Part print with two shaded views. Sizes in mm from the minimum x, y, z corner. Give positions to 0.01 mm unless a question says otherwise; leave off trailing zeros. Order: outer loops, then holes, each group sorted by start corner. A loop starts at its lowest first (then second) coordinate and runs counter-clockwise, first axis right, second up. Notation, with made-up numbers: M 25,-3 L 48,-3 A25 ccw 48,29 Z; hole C 78,78 d5. An arc over 180 degrees is marked long. Return JSON: item names as keys, results as strings.
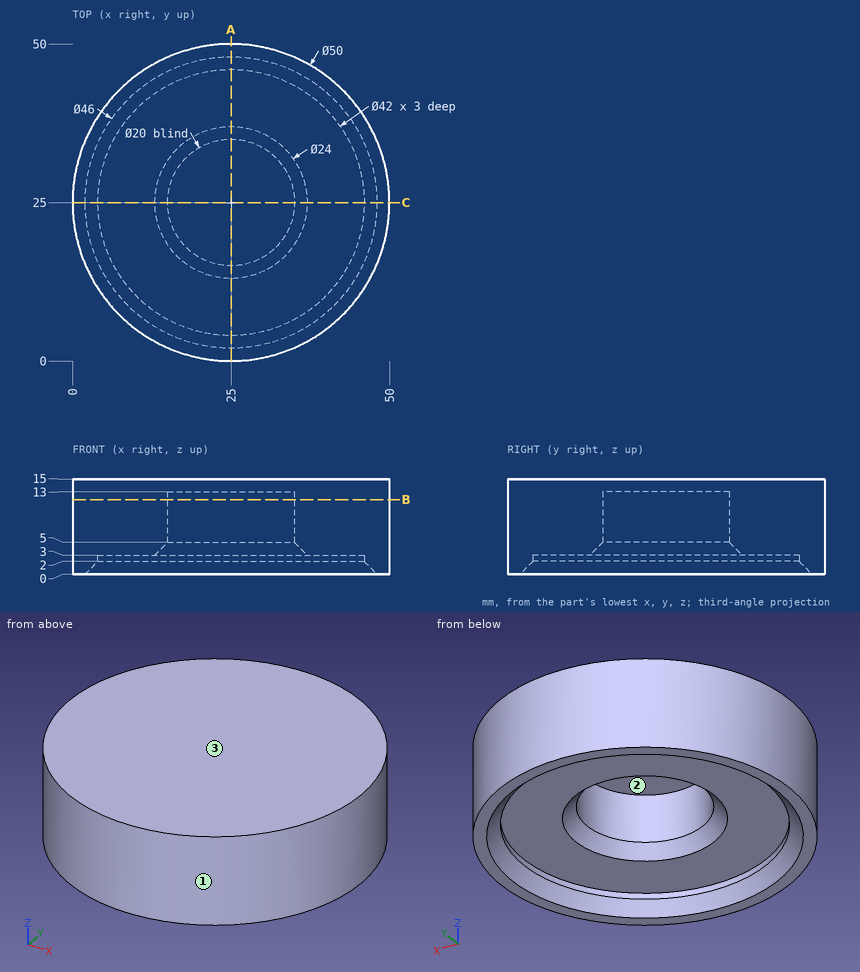
Q1. Probe line 1 along Y through (x, z) = (25, 9.25); line 2 along Z through (x, y) = (12.5, 35); line 3 along Y through (x, z) = (25, 2.7). List the from-to ranges inside material, lowest first.
Established:
{"line 1": "y = 0 to 15, 35 to 50", "line 2": "z = 3 to 15", "line 3": "y = 0 to 4, 46 to 50"}
Q2. Pin check, flat tips, straight feed: pin 1 (6 mm diameter, centred on y = 45, z = 6, fed in from -X); pin 2 (1.5 mm diameter, centred on x = 40, z = 10, fed in from +Y); pin 3 (6 mm diameter, centred on y = 30.5, z = 1.5, fed in from -X). Stop position of each tip, or through.
Established:
{"pin 1": "stops at x = 6.67", "pin 2": "stops at y = 45.54", "pin 3": "stops at x = 0.13"}
Q3. Band-saw the part on A-A (x = 25). Give the cut face in (y, z).
Established:
{"outline": "M 0,0 L 2,0 L 4,2 L 4,3 L 13,3 L 15,5 L 15,13 L 35,13 L 35,5 L 37,3 L 46,3 L 46,2 L 48,0 L 50,0 L 50,15 L 0,15 Z"}
Q4. Two-plate mould, pull along X, no slides. Class the marked faces 1, 2 and 3: +X half, -X half, draft (parallel to the pull), parting line (faces both ways), or undercut.
Established:
{"face 1": "parting line", "face 2": "undercut", "face 3": "draft"}
Q5. Band-saw the part on B-B (z = 11.75). Give the cut face in (x, y), then the cut area to 3 significant figures.
Established:
{"outline": "C 25,25 d50; hole C 25,25 d20", "area": "1,650 mm²"}
